from build123d import *

# Parameters (mm, degrees)
BOSS_EXTRUDE1_OUTLINE_R = 3.9500048
BOSS_EXTRUDE1_DEPTH     = 8.5875
BOSS_EXTRUDE2_START     = -1.5875
SKETCH4_R               = 6
SKETCH4_R_2             = 3.9500048
BOSS_EXTRUDE2_DEPTH     = 1.5875


# Read off the part's stored shape, not the designer's step: Boss-Extrude1
with BuildPart() as part:
    # Boss-Extrude1 outline → Boss-Extrude1 (new body)
    with BuildSketch(Plane.XY):
        Circle(BOSS_EXTRUDE1_OUTLINE_R)
        with BuildLine():
            Line((2.067410216, -3.2385), (-2.067410216, -3.2385))
            ThreePointArc((-2.067410216, -3.2385), (-2.123342942, -3.230103762), (-2.174345227, -3.205655172))
            ThreePointArc((-2.174345227, -3.205655172), (-2.738978117, -2.738978117), (-3.205655172, -2.174345227))
            ThreePointArc((-3.205655172, -2.174345227), (-3.230103762, -2.123342942), (-3.2385, -2.067410216))
            Line((-3.2385, -2.067410216), (-3.2385, 2.067410216))
            ThreePointArc((-3.2385, 2.067410216), (-3.230103762, 2.123342942), (-3.205655172, 2.174345227))
            ThreePointArc((-3.205655172, 2.174345227), (-2.738978117, 2.738978117), (-2.174345227, 3.205655172))
            ThreePointArc((-2.174345227, 3.205655172), (-2.123342942, 3.230103762), (-2.067410216, 3.2385))
            Line((-2.067410216, 3.2385), (2.067410216, 3.2385))
            ThreePointArc((2.067410216, 3.2385), (2.123342942, 3.230103762), (2.174345227, 3.205655172))
            ThreePointArc((2.174345227, 3.205655172), (2.738978117, 2.738978117), (3.205655172, 2.174345227))
            ThreePointArc((3.205655172, 2.174345227), (3.230103762, 2.123342942), (3.2385, 2.067410216))
            Line((3.2385, 2.067410216), (3.2385, -2.067410216))
            ThreePointArc((3.2385, -2.067410216), (3.230103762, -2.123342942), (3.205655172, -2.174345227))
            ThreePointArc((3.205655172, -2.174345227), (2.738978117, -2.738978117), (2.174345227, -3.205655172))
            ThreePointArc((2.174345227, -3.205655172), (2.123342942, -3.230103762), (2.067410216, -3.2385))
        make_face(mode=Mode.SUBTRACT)
    extrude(amount=BOSS_EXTRUDE1_DEPTH)

    # Sketch4 → Boss-Extrude2 (add)
    with BuildSketch(Plane.XY.offset(8.5875).offset(BOSS_EXTRUDE2_START)):
        Circle(SKETCH4_R)
        Circle(SKETCH4_R_2, mode=Mode.SUBTRACT)
    extrude(amount=BOSS_EXTRUDE2_DEPTH)


solid = part.part
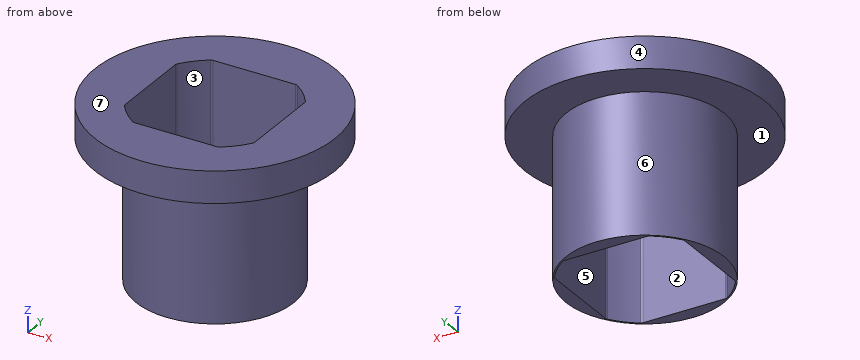
Here's how the part is built. I have some questions about the finished solid (model axes, mm). Face numbers are marked on the shaded views. A direction names the side the tool comes from. Round coordinates to 2 decimals unless told otherwise and drop trailing zeros. Order: outer loops, then holes, each group sorted by start corner. A loop starts at its lowest first (then second) coordinate and runs counter-clockwise, first axis right, second up. Notation, with made-up numbers: (60, 48) -> (79, 48) arc R25 cw to (79, 66) -> close; hole circle Ø1 at (-34.75, -36.5). An arc over 180 degrees is marked (long way). Return JSON: item names as keys, results as strings.
Q1. If we mould it in two halves opening along X, with no side actions, what happens to the marked faces 1, 2, 3 and 4? For each: released by +X, released by -X, zero draft, split by the parting line, or undercut.
Filled sheet:
{"face 1": "zero draft", "face 2": "undercut", "face 3": "undercut", "face 4": "split by the parting line"}
Q2. I need wall thicknesses on line 1 along Z through (x, y) = (0.5, 4.25); line 2 along X through (y, z) = (0.5, 8); line 3 along Y through (x, z) = (0.75, 1.25). Which ranges of each line are inside material? Lowest first, please. Write a range as from..to.
Filled sheet:
{"line 1": "z = 7..8.59", "line 2": "x = -5.98..-3.24, 3.24..5.98", "line 3": "y = -3.88..-3.24, 3.24..3.88"}
Q3. If we section it at D-D on z = 8: List the corners of the cut face in (x, y) for me, plus the area to 3 significant figures.
Filled sheet:
{"outline": "circle Ø12 at (0, 0); hole (-3.24, -2.07) arc R0.19 ccw to (-3.21, -2.17) arc R3.87 ccw to (-2.17, -3.21) arc R0.19 ccw to (-2.07, -3.24) -> (2.07, -3.24) arc R0.19 ccw to (2.17, -3.21) arc R3.87 ccw to (3.21, -2.17) arc R0.19 ccw to (3.24, -2.07) -> (3.24, 2.07) arc R0.19 ccw to (3.21, 2.17) arc R3.87 ccw to (2.17, 3.21) arc R0.19 ccw to (2.07, 3.24) -> (-2.07, 3.24) arc R0.19 ccw to (-2.17, 3.21) arc R3.87 ccw to (-3.21, 2.17) arc R0.19 ccw to (-3.24, 2.07) -> close", "area": "73.3 mm^2"}
Q4. If we section it at A-A on x = 0: List the corners of the cut face in (y, z) for me, plus the area to 3 significant figures.
Filled sheet:
{"outline": "(-6, 7) -> (-3.95, 7) -> (-3.95, 0) -> (-3.24, 0) -> (-3.24, 8.59) -> (-6, 8.59) -> close; (3.24, 0) -> (3.95, 0) -> (3.95, 7) -> (6, 7) -> (6, 8.59) -> (3.24, 8.59) -> close", "area": "18.7 mm^2"}
Q5. If we section it at C-C on z = 1.25: List the corners of the cut face in (x, y) for me, plus the area to 3 significant figures.
Filled sheet:
{"outline": "circle Ø7.9 at (0, 0); hole (-3.24, -2.07) arc R0.19 ccw to (-3.21, -2.17) arc R3.87 ccw to (-2.17, -3.21) arc R0.19 ccw to (-2.07, -3.24) -> (2.07, -3.24) arc R0.19 ccw to (2.17, -3.21) arc R3.87 ccw to (3.21, -2.17) arc R0.19 ccw to (3.24, -2.07) -> (3.24, 2.07) arc R0.19 ccw to (3.21, 2.17) arc R3.87 ccw to (2.17, 3.21) arc R0.19 ccw to (2.07, 3.24) -> (-2.07, 3.24) arc R0.19 ccw to (-2.17, 3.21) arc R3.87 ccw to (-3.21, 2.17) arc R0.19 ccw to (-3.24, 2.07) -> close", "area": "9.21 mm^2"}
Q6. Which directions (+Z, -Z, +X, -X, +Y, -Y) give clear straight access to the entire face, cutting with the end or side of a thin tool? Please do the marked faces 5, 6 and 7.
Filled sheet:
{"face 5": "+Z, -Z", "face 6": "-Z", "face 7": "+Z, +X, -X, +Y, -Y"}
Q7. For pin 1 Ø1.2 at (x, z) = (0.5, 6) entering from +Y; pin 2 Ø3 at (x, z) = (4, 6.5) entering from -Y; pin 3 Ø5 at (y, z) = (-2.5, 2.5) entering from -X; pin 4 Ø2 at (x, y) = (-1, -2) entering from -Z, each with a flat end and sliding along its axis, tell me the tip position at first contact or that it passes through.
Filled sheet:
{"pin 1": "stops at y = 3.95", "pin 2": "stops at y = -5.41", "pin 3": "stops at x = -3.95", "pin 4": "passes through"}
